```python
from build123d import *

# Parameters (mm, degrees)
BOSS_EXTRUDE1_DEPTH = 5
FILLET1_R           = 3
FILLET2_R           = 2


with BuildPart() as part:
    # Sketch2 → Boss-Extrude1 (new body)
    with BuildSketch(Plane(origin=(0, 0, 0), x_dir=(1, 0, 0), z_dir=(0, 1, 0))):
        Polygon((0, 0), (0, 60.1), (33, 60.1), (33, 0), (25.030442415, 0.697245942), (24.812553058, -1.793240803), (35.5, -2.728271253), (35.5, 62.6), (-2.5, 62.6), (-2.5, -2.728271253), (8.187446942, -1.793240803), (7.969557585, 0.697245942), align=None)
    extrude(amount=BOSS_EXTRUDE1_DEPTH)

    # Fillet1
    fillet1_edges = [part.edges().sort_by_distance(p)[0] for p in [
        (33, 2.5, -60.1),
        (0, 2.5, -60.1),
    ]]
    fillet(fillet1_edges, radius=FILLET1_R)

    # Fillet2
    fillet2_edges = [part.edges().sort_by_distance(p)[0] for p in [
        (8.187446942, 2.5, 1.793240803),
        (-2.5, 2.5, 2.728271253),
        (-2.5, 2.5, -62.6),
        (35.5, 2.5, -62.6),
        (35.5, 2.5, 2.728271253),
        (24.812553058, 2.5, 1.793240803),
    ]]
    fillet(fillet2_edges, radius=FILLET2_R)


solid = part.part
```
Can you work these out from the model? Positions are in its coordinate system, mm. A direction names the side the tool comes from. Give positions to 0.01 mm unless a question says otherwise; leave off trailing zeros. Order: outer loops, then holes, each group sorted by start corner. A loop starts at its lowest first (then second) coordinate and runs counter-clockwise, first axis right, second up. Notation, with made-up numbers: M 20,-40 L 70,-40 A19 cw 70,-17 Z; hole C -6.75,39.25 d8. An arc over 180 degrees is marked long. Write item = value, one per line. Start each with the question number.
Q1. I need wall thicknesses on probe 1 along X at (y, z) = (2.2, -12.5); probe 2 along Z at (x, y) = (18.5, 3.65); probe 3 along Z at (x, y) = (26, 3.55). Which ranges of each line are inside material? Lowest first, please. Write a range as [from, to].
Q2. We'd pull the mould along X, two halves only. Please class faces 1 (the flat face through (35.5, 2, -30)), 2 (the flat face through (-0.5, 5, -35)), 3 (the cylindrical face through (0.86, 2.54, -59.2)): pulls with the +X half, pulls with the -X half, needs draft (parallel to the pull), parting line crosses it, or undercut.
Q3. For faces 4 (the flat face through (-2.5, 2, -30)), 5 (the flat face through (2.889, 2.465, 2.257)), 6 (the flat face through (0, 2, -28)), which set-ups out of +Z, -Z, +X, -X, +Y, -Y let a thin tool reach every point of the face, with its end or its side?
Q4. Suppose I cut it at C-C (x = 26). Write out the boundary of the cut face in (y, z).
Q5. Suppose I cut it at D-D (x = 20). Write out the boundary of the cut face in (y, z).
Q6. Suppose I cut it at A-A (z = -19). Write out the boundary of the cut face in (x, y).
Q7. Suppose I cut it at B-B (y = 3.1). Write out the boundary of the cut face in (x, z), plus the area to 3 significant figures.
Check result:
q1.probe_1 = [-2.5, 0], [33, 35.5]
q1.probe_2 = [-62.6, -60.1]
q1.probe_3 = [-62.6, -60.1], [-0.61, 1.72]
q2.face_1 = pulls with the +X half
q2.face_2 = needs draft
q2.face_3 = undercut
q3.face_4 = +Z, -Z, -X, +Y, -Y
q3.face_5 = +Z, +Y, -Y
q3.face_6 = +Y, -Y
q4.outline = M 0,-62.6 L 5,-62.6 L 5,-60.1 L 0,-60.1 Z; M 0,-0.61 L 5,-0.61 L 5,1.72 L 0,1.72 Z
q5.outline = M 0,-62.6 L 5,-62.6 L 5,-60.1 L 0,-60.1 Z
q6.outline = M -2.5,0 L 0,0 L 0,5 L -2.5,5 Z; M 33,0 L 35.5,0 L 35.5,5 L 33,5 Z
q7.outline = M -2.5,-60.6 A2 ccw -0.5,-62.6 L 33.5,-62.6 A2 ccw 35.5,-60.6 L 35.5,0.55 A2 ccw 33.33,2.54 L 26.8,1.97 A2 ccw 24.99,-0.2 L 25.03,-0.7 L 33,0 L 33,-57.1 A3 cw 30,-60.1 L 3,-60.1 A3 cw 0,-57.1 L 0,0 L 7.97,-0.7 L 8.01,-0.2 A2 ccw 6.2,1.97 L -0.33,2.54 A2 ccw -2.5,0.55 Z
q7.area = 447 mm2
